```python
from build123d import *

# Parameters (mm, degrees)
BOSS_EXTRUDE3_DEPTH = 65
BOSS_EXTRUDE4_REACH = 153.013
SKETCH4_W           = 128
SKETCH4_H           = 2
SKETCH5_W           = 12
SKETCH5_H           = 53.559358602
CUT_EXTRUDE2_DEPTH  = 11
FILLET1_R           = 5
FILLET2_R           = 2
SKETCH7_W           = 90
SKETCH7_H           = 61
BOSS_EXTRUDE5_DEPTH = 2
BOSS_EXTRUDE6_DEPTH = 5
SKETCH12_R          = 1.5
CUT_EXTRUDE5_DEPTH  = 20
BOSS_EXTRUDE7_START = 13
BOSS_EXTRUDE7_DEPTH = 13
SKETCH15_R          = 1.5
CUT_EXTRUDE6_DEPTH  = 21
SKETCH16_W          = 6.5
SKETCH16_H          = 61
CUT_EXTRUDE7_DEPTH  = 2
FILLET3_R           = 3
FILLET4_R           = 3
CUT_EXTRUDE9_DEPTH  = 2
SKETCH18_W          = 6.5
SKETCH18_H          = 37.103743482
BOSS_EXTRUDE8_DEPTH = 2


with BuildPart() as part:
    # Sketch3 → Boss-Extrude3 (new body)
    with BuildSketch(Plane(origin=(0, 0, 0), x_dir=(1, 0, 0), z_dir=(0, 1, 0))):
        Polygon((0, 0), (0, 25), (-2, 25), (-2, 2), (-92, 2), (-130, -6.55), (-130, 25), (-132, 25), (-132, -9), (-92, 0), align=None)
    extrude(amount=BOSS_EXTRUDE3_DEPTH)

    # Sketch4 → Boss-Extrude4 (add, up to next)
    with BuildSketch(Plane(origin=(0, 0, -25), x_dir=(-1, 0, 0), z_dir=(0, 0, -1)), mode=Mode.PRIVATE) as boss_extrude4_sk1:
        with Locations((66, 64)):
            Rectangle(SKETCH4_W, SKETCH4_H)
    boss_extrude4_tool1 = extrude(boss_extrude4_sk1.sketch, amount=-BOSS_EXTRUDE4_REACH, mode=Mode.PRIVATE) - part.part
    # Sketch4 → Boss-Extrude4 (add, up to next)
    with BuildSketch(Plane(origin=(0, 0, -25), x_dir=(-1, 0, 0), z_dir=(0, 0, -1)), mode=Mode.PRIVATE) as boss_extrude4_sk2:
        with Locations((66, 1)):
            Rectangle(SKETCH4_W, SKETCH4_H)
    boss_extrude4_tool2 = extrude(boss_extrude4_sk2.sketch, amount=-BOSS_EXTRUDE4_REACH, mode=Mode.PRIVATE) - part.part
    add(boss_extrude4_tool1.solids().sort_by_distance((-66, 64, -25))[0])
    add(boss_extrude4_tool2.solids().sort_by_distance((-66, 1, -25))[0])

    # Sketch5 → Cut-Extrude2 (cut)
    with BuildSketch(Plane.ZY.offset(132)):
        with Locations((-14, 32.5)):
            Rectangle(SKETCH5_W, SKETCH5_H)
    extrude(amount=-CUT_EXTRUDE2_DEPTH, mode=Mode.SUBTRACT)

    # Fillet1
    fillet1_edges = [part.edges().sort_by_distance(p)[0] for p in [
        (-132, 32.5, 9),
    ]]
    fillet(fillet1_edges, radius=FILLET1_R)

    # Fillet2
    fillet2_edges = [part.edges().sort_by_distance(p)[0] for p in [
        (-132, 0, -11.125),
        (-46, 0, 0),
        (-92, 32.5, 0),
        (0, 32.5, 0),
        (-132, 65, -11.125),
        (-46, 65, 0),
        (-108.951219512, 0, 3.81402439),
        (-108.951219512, 65, 3.81402439),
        (-130.123475238, 0, 6.654344047),
        (-130.123475238, 65, 6.654344047),
    ]]
    fillet(fillet2_edges, radius=FILLET2_R)

    # Sketch7 → Boss-Extrude5 (add)
    with BuildSketch(Plane(origin=(0, 0, -2), x_dir=(-1, 0, 0), z_dir=(0, 0, -1))):
        with Locations((47, 32.5)):
            Rectangle(SKETCH7_W, SKETCH7_H)
    extrude(amount=BOSS_EXTRUDE5_DEPTH)

    # Sketch11 → Boss-Extrude6 (add)
    with BuildSketch(Plane(origin=(0, 0, -25), x_dir=(-1, 0, 0), z_dir=(0, 0, -1))):
        with BuildLine():
            Line((7, 63), (2, 63))
            Line((2, 63), (2, 58))
            ThreePointArc((2, 58), (5.535533906, 59.464466094), (7, 63))
        make_face()
        with BuildLine():
            Line((2, 7), (2, 2))
            Line((2, 2), (7, 2))
            ThreePointArc((7, 2), (5.535533906, 5.535533906), (2, 7))
        make_face()
        with BuildLine():
            Line((125, 2), (130, 2))
            Line((130, 2), (130, 7))
            ThreePointArc((130, 7), (126.464466094, 5.535533906), (125, 2))
        make_face()
        with BuildLine():
            Line((125, 63), (130, 63))
            Line((130, 63), (130, 58))
            ThreePointArc((130, 58), (126.464466094, 59.464466094), (125, 63))
        make_face()
    extrude(amount=-BOSS_EXTRUDE6_DEPTH)

    # Sketch12 → Cut-Extrude5 (cut)
    with BuildSketch(Plane(origin=(0, 0, -25), x_dir=(-1, 0, 0), z_dir=(0, 0, -1))):
        with Locations((3.767766953, 61.232233047)):
            Circle(SKETCH12_R)
        with Locations((128.232233047, 61.232233047)):
            Circle(SKETCH12_R)
        with Locations((128.232233047, 3.767766953)):
            Circle(SKETCH12_R)
        with Locations((3.767766953, 3.767766953)):
            Circle(SKETCH12_R)
    extrude(amount=-CUT_EXTRUDE5_DEPTH, mode=Mode.SUBTRACT)

    # Sketch14 → Boss-Extrude7 (add)
    with BuildSketch(Plane(origin=(0, 0, -4), x_dir=(-1, 0, 0), z_dir=(0, 0, -1)).offset(BOSS_EXTRUDE7_START)):
        with BuildLine():
            Line((2, 58), (2, 63))
            Line((2, 63), (7, 63))
            ThreePointArc((7, 63), (5.535533906, 59.464466094), (2, 58))
        make_face()
        with BuildLine():
            Line((2, 2), (7, 2))
            ThreePointArc((7, 2), (5.535533906, 5.535533906), (2, 7))
            Line((2, 7), (2, 2))
        make_face()
    extrude(amount=-BOSS_EXTRUDE7_DEPTH)

    # Sketch15 → Cut-Extrude6 (cut)
    with BuildSketch(Plane(origin=(0, 0, -25), x_dir=(-1, 0, 0), z_dir=(0, 0, -1))):
        with Locations((3.767766953, 3.767766953)):
            Circle(SKETCH15_R)
        with Locations((3.767766953, 61.232233047)):
            Circle(SKETCH15_R)
    extrude(amount=-CUT_EXTRUDE6_DEPTH, mode=Mode.SUBTRACT)

    # Sketch16 → Cut-Extrude7 (cut)
    with BuildSketch(Plane(origin=(0, 0, -4), x_dir=(-1, 0, 0), z_dir=(0, 0, -1))):
        with Locations((59.5, 32.5)):
            Rectangle(SKETCH16_W, SKETCH16_H)
    extrude(amount=-CUT_EXTRUDE7_DEPTH, mode=Mode.SUBTRACT)

    # Fillet3
    # the kernel refuses this fillet: 3 mm, written as the material it adds along each edge
    with BuildSketch(Plane(origin=(-92, 2, -2), x_dir=(-2.9487523534032267e-12, 0, -1.0), z_dir=(0, 1, 0))) as fillet3_piece_1:
        with BuildLine():
            CenterArc((2.406216573, 2.972370787), FILLET3_R, 192.680383492, 69.537546468)
            Line((-0.520612695, 2.313834202), (-0.579149281, 2.30066347))
            Line((-0.579149281, 2.30066347), (-0.058536585, -0.013170732))
            Line((-0.058536585, -0.013170732), (0, -0.06))
            ThreePointArc((0, -0.06), (1, -0.06), (1.991875669, -0.059447416))
            Line((1.991875669, -0.059447416), (2, 0))
        make_face()
    extrude(amount=61)

    # Fillet4
    fillet4_edges = [part.edges().sort_by_distance(p)[0] for p in [
        (-92, 32.5, -4),
    ]]
    fillet(fillet4_edges, radius=FILLET4_R)

    # Sketch17 → Cut-Extrude9 (cut)
    with BuildSketch(Plane(origin=(0, 0, -2), x_dir=(-1, 0, 0), z_dir=(0, 0, -1))):
        Polygon((59.5, 53), (61.5, 53), (61.5, 63), (57.5, 63), (57.5, 53), align=None)
        Polygon((57.5, 2), (61.5, 2), (61.5, 12), (59.5, 12), (57.5, 12), align=None)
    extrude(amount=-CUT_EXTRUDE9_DEPTH, mode=Mode.SUBTRACT)

    # Sketch18 → Boss-Extrude8 (add)
    with BuildSketch(Plane(origin=(0, 0, -2), x_dir=(-1, 0, 0), z_dir=(0, 0, -1))):
        with Locations((59.5, 32.5)):
            Rectangle(SKETCH18_W, SKETCH18_H)
    extrude(amount=BOSS_EXTRUDE8_DEPTH)


solid = part.part
```
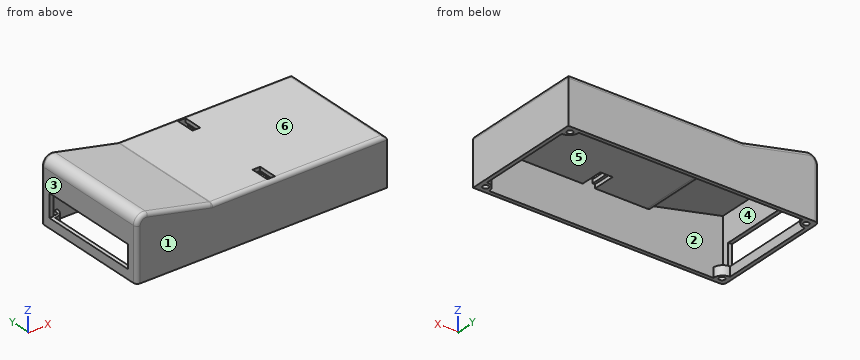
Input: part model. Units: mm. Frame: model coordinates. Face numbers are marked on the shaded views. A direction names the side the tool comes from. Give positions to 0.01 mm unless a question says otherwise; leave off trailing zeros. Loops run counter-clockwise (first coordinate to the right, second up) from the corner with the lowest first, then second, coordinate; pieces in that order, holes last. Notation, with made-up numbers: M -27.75,2 L -16.75,2 A32 ccw -16.75,37 Z; hole C 42,42 d11. An arc over 180 degrees is marked long. Answer as CSV lines item,"result". Start each with the question number.
1. Section A-A on y = 34. Return loops of the section in (x, z), plus the area to 3 significant figures.
2. Line query: L1, parallel to Y at x = -8, z = -12.5; L2, parallel to X at y = 33, z = -22; L3, parallel to X at y = 49, z = -11. Output: solid intervals per line, ascending.
3. Section B-B on z = -23. Return loops of the section in (x, y), plus the area to 3 significant figures.
4. Pin query (flat end, axial travel): P1, Ø2, axis at x = -60, y = 9.5, coming from the -Z side; P2, Ø10.5, axis at y = 17.5, z = -11, coming from the -X side; P3, Ø10, axis at x = -106, y = 10, coming from the +Z side (3 decimals); P4, Ø2.5, axis at x = -3.77, y = 61.23, coming from the +Z side. Return the tip coordinate at first contact, or that it passes through.
5. Pull-direction query (Y, two-part tool) for the marked faces 1, 2 and 3; classes: released by +Y, released by -Y, zero draft, split by the parting line, or undercut.
6. Section C-C on x = -45.5. Return loops of the section in (y, z), plus the area to 3 significant figures.
7. Reachability of the marked faces 4, 5 and 6 from +Z, -Z, +X, -X, +Y, -Y: full face, straight path, thin tool, end or side. Return the list, or none.
8. Section D-D on z = -11. Return loops of the section in (x, y).
Computed values:
1,outline,"M -132,-25 L -130,-25 L -130,-20 L -132,-20 Z; M -132,-8 L -130,-8 L -130,6.55 L -94.31,-1.48 A3 cw -92.5,-2.7 A3 ccw -90.03,-4 L -2,-4 L -2,-25 L 0,-25 L 0,-2 A2 ccw -2,0 L -91.78,0 A2 cw -92.22,0.05 L -125.9,7.63 A5 ccw -132,2.75 Z"
1,area,"520 mm²"
2,L1,"y = 0 to 2, 63 to 65"
2,L2,"x = -132 to -130, -2 to 0"
2,L3,"x = -2 to 0"
3,outline,"M -132,2 A2 ccw -130,0 L 0,0 L 0,65 L -130,65 A2 ccw -132,63 Z; hole M -130,7 A5 cw -125,2 L -7,2 A5 cw -2,7 L -2,58 A5 cw -7,63 L -125,63 A5 cw -130,58 Z; hole C -128.23,3.77 d3; hole C -128.23,61.23 d3; hole C -3.77,3.77 d3; hole C -3.77,61.23 d3"
3,area,"821 mm²"
4,P1,"passes through"
4,P2,"stops at x = -132"
4,P3,"stops at z = 4.275"
4,P4,"stops at z = 0"
5,face 1,"released by -Y"
5,face 2,"undercut"
5,face 3,"zero draft"
6,outline,"M 0,-25 L 2,-25 L 2,-4 L 63,-4 L 63,-25 L 65,-25 L 65,-2 A2 ccw 63,0 L 2,0 A2 ccw 0,-2 Z"
6,area,"342 mm²"
7,face 4,"none"
7,face 5,"-Z"
7,face 6,"+Z, +X, +Y, -Y"
8,outline,"M -132,2 A2 ccw -130,0 L 0,0 L 0,65 L -130,65 A2 ccw -132,63 L -132,59.28 L -130,59.28 L -130,63 L -7,63 A5 ccw -2,58 L -2,7 A5 ccw -7,2 L -130,2 L -130,5.72 L -132,5.72 Z; hole C -3.77,3.77 d3; hole C -3.77,61.23 d3"
